The listing builds one solid part. Answer for the finished solid, in the listing's coordinates (mm). Coordinates: 2 decimals unless noted, no trailing zeros. Loops run counter-clockwise (first coordinate to the right, second up) from the corner with the lowest first, then second, coordinate; pieces in that order, holes last. Notation, with made-up numbers: M 1,87 L 50,87 A19 cw 50,104 Z; hole C 68,27.5 d2. An arc over 180 degrees is marked long. Return JSON: item names as keys, results as strings. Group by question number.
1. Given P1, Ø1.5, axis at x = 2, z = -207.5, coming from the +Y side, flat-ended and moving along its own axis, determine where the tip first touches the part or whether it passes through.
2. Section C-C (z = -186) is taken. Write down the section's boundary in (x, y), then the cut area to 3 significant figures.
3. Section A-A (y = -3) is taken. Write down the section's boundary in (x, z), then the cut area to 3 significant figures.
4. Section D-D (z = 55.5) is taken. Write down the section's boundary in (x, y).
5. Straight lines are drawn through the part: L1, parallel to Z at x = 2.05, y = 0.5; L2, parallel to Z at x = 1, y = -11.5; L3, parallel to Y at x = 0.6, z = 29. For each, find the intervals that lie inside material, in ascending order. Write a range as from..to.
```python
from build123d import *

# Parameters (mm, degrees)
BOSS_EXTRUDE1_DEPTH = 5


with BuildPart() as part:
    # Sketch1 → Boss-Extrude1 (new body)
    with BuildSketch(Plane(origin=(0, 0, 0), x_dir=(0, 0, -1), z_dir=(1, 0, 0))):
        Polygon((-247, 67.5), (-148.2, 67.5), (-148.2, 72.5), (-49.4, 72.5), (-49.4, 67.5), (49.4, 67.5), (49.4, 72.5), (148.2, 72.5), (148.2, 67.5), (247, 67.5), (247, -72.5), (141.262721236, -72.5), (141.262721236, -56.5), (136.262721236, -56.5), (136.262721236, -40.5), (141.262721236, -40.5), (141.262721236, -24.5), (136.262721236, -24.5), (136.262721236, -8.5), (141.262721236, -8.5), (141.262721236, 7.5), (0, 7.5), (-137.5, 7.5), (-137.5, -8.5), (-142.5, -8.5), (-142.5, -24.5), (-137.5, -24.5), (-137.5, -40.359311741), (-142.5, -40.5), (-142.5, -56.5), (-137.5, -56.5), (-137.5, -72.5), (-247, -72.5), align=None)
    extrude(amount=BOSS_EXTRUDE1_DEPTH)


solid = part.part
```
Worked out:
{
 "1": {"P1": "y = 67.5"},
 "2": {"outline": "M 0,-72.5 L 5,-72.5 L 5,67.5 L 0,67.5 Z", "area": "700 mm^2"},
 "3": {"outline": "M 0,-247 L 5,-247 L 5,-141.26 L 0,-141.26 Z; M 0,137.5 L 5,137.5 L 5,247 L 0,247 Z", "area": "1,080 mm^2"},
 "4": {"outline": "M 0,7.5 L 5,7.5 L 5,72.5 L 0,72.5 Z"},
 "5": {"L1": "-247..-141.26, 137.5..247", "L2": "-247..-136.26, 142.5..247", "L3": "7.5..67.5"}
}
